from build123d import *

# Parameters (mm, degrees)
BASE_FLANGE1_DEPTH    = 10
FILLET1_R             = 3
SKETCH7_R             = 1.5
SKETCH7_R_2           = 1
CUT_EXTRUDE1_DEPTH    = 39.303728604
BODY_MOVE_COPY1_ANGLE = 90


# Sheet-metal steps are written as plain solids
with BuildPart() as part:
    # Sketch1 → Base-Flange1 (new, symmetric)
    with BuildSketch(Plane.XY):
        with BuildLine():
            Line((-12, 0), (-2.75, 0))
            ThreePointArc((-2.75, 0), (-0.805456352, 0.805456352), (0, 2.75))
            Line((0, 2.75), (0, 15.775))
            ThreePointArc((0, 15.775), (0.219669914, 16.305330086), (0.75, 16.525))
            Line((0.75, 16.525), (32, 16.525))
            Line((32, 16.525), (32, 18.525))
            Line((32, 18.525), (0.75, 18.525))
            ThreePointArc((0.75, 18.525), (-1.194543648, 17.719543648), (-2, 15.775))
            Line((-2, 15.775), (-2, 2.75))
            ThreePointArc((-2, 2.75), (-2.219669914, 2.219669914), (-2.75, 2))
            Line((-2.75, 2), (-12, 2))
            Line((-12, 2), (-12, 0))
        make_face()
    extrude(amount=BASE_FLANGE1_DEPTH, both=True)

    # Fillet1
    fillet1_edges = [part.edges().sort_by_distance(p)[0] for p in [
        (32, 17.525, -10),
        (-12, 1, -10),
        (32, 17.525, 10),
        (-12, 1, 10),
    ]]
    fillet(fillet1_edges, radius=FILLET1_R)

    # Sketch7 → Cut-Extrude1 (cut, through all)
    with BuildSketch(Plane(origin=(0, 0, 0), x_dir=(1, 0, 0), z_dir=(0, 1, 0))):
        with Locations((-9, 6)):
            Circle(SKETCH7_R)
        with Locations((-9, -6)):
            Circle(SKETCH7_R)
        with Locations(Location((14.875, 0, 0), (0, 0, 90))):
            Circle(SKETCH7_R_2)
    extrude(amount=CUT_EXTRUDE1_DEPTH, mode=Mode.SUBTRACT)


with BuildPart() as part_1:
    # Body-Move/Copy1: moved
    add(part.part.rotate(Axis((0, 7.6, 0), (1, 0, 0)), BODY_MOVE_COPY1_ANGLE))


solid = part_1.part
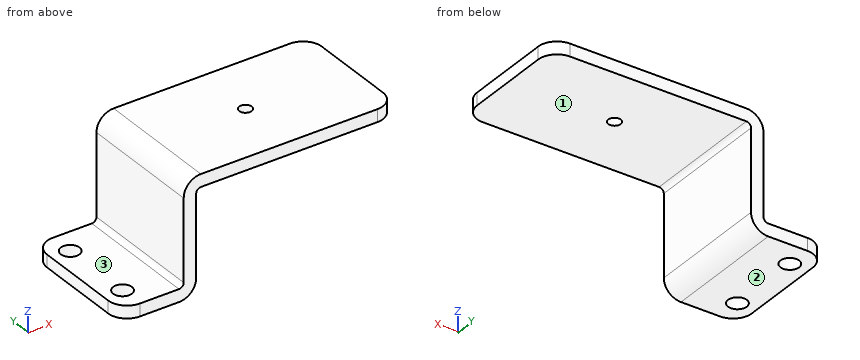
Can you work these out from the model? Positions are in its coordinate system, mm. Face numbers are marked on the shaded views. A direction names the side the tool comes from. Coordinates: 2 decimals unless noted, no trailing zeros. Write each loop counter-clockwise with the first axis right and the second up, starting at its lowest first coordinate (ties: lowest second). Pieces come first, ordered by that corner, then holes.
Q1. For P1, Ø4, axis at x = 22, y = 4, coming from the -Z side (3 decimals); P2, Ø10.5, axis at y = 10.5, z = 0, coming from the -X side; P3, Ø4, axis at y = 6.5, z = 5, coming from the +X side, each with a flat end and sliding along its axis, tell me the tip position at first contact or that it passes through.
Results found:
P1: stops at z = 8.925
P2: stops at x = -2.12
P3: stops at x = 0
Q2. Imagine slicing it at D-D, the plane x = 3. List the corners of the cut face in (y, z) for me (3 decimals).
Results found:
outline: (-2.4, 8.925) - (17.6, 8.925) - (17.6, 10.925) - (-2.4, 10.925) - close
Q3. Please list where these lines run through material, in increasing order: L1, parallel to Y at x = -9, z = -5.95; L2, parallel to X at y = 6.75, z = 0.75; L3, parallel to Z at x = -4, y = 8.
Results found:
L1: y = -2.4 to 0.1, 3.1 to 12.1, 15.1 to 17.6
L2: x = -2 to 0
L3: z = -7.6 to -5.6
Q4. Imagine slicing it at B-B, the plane y = 1.6. List the corners of the cut face in (x, z) for me (3 decimals).
Results found:
outline: (-12, -7.6) - (-10.5, -7.6) - (-10.5, -5.6) - (-12, -5.6) - close; (-7.5, -7.6) - (-2.75, -7.6) arc R2.75 ccw to (0, -4.85) - (0, 8.175) arc R0.75 cw to (0.75, 8.925) - (32, 8.925) - (32, 10.925) - (0.75, 10.925) arc R2.75 ccw to (-2, 8.175) - (-2, -4.85) arc R0.75 cw to (-2.75, -5.6) - (-7.5, -5.6) - close
Q5. Imagine slicing it at C-C, the plane z = 6. List the corners of the cut face in (x, y) for me.
Results found:
outline: (-2, -2.4) - (0, -2.4) - (0, 17.6) - (-2, 17.6) - close
Q6. Imagine slicing it at A-A, the plane y = 7.6. List the corners of the cut face in (x, z) for me (3 decimals).
Results found:
outline: (-12, -7.6) - (-2.75, -7.6) arc R2.75 ccw to (0, -4.85) - (0, 8.175) arc R0.75 cw to (0.75, 8.925) - (13.875, 8.925) - (13.875, 10.925) - (0.75, 10.925) arc R2.75 ccw to (-2, 8.175) - (-2, -4.85) arc R0.75 cw to (-2.75, -5.6) - (-12, -5.6) - close; (15.875, 8.925) - (32, 8.925) - (32, 10.925) - (15.875, 10.925) - close
Q7. Which directions (+Z, -Z, +X, -X, +Y, -Y) give clear straight access to the entire face, cutting with the end or side of a thin tool? Please do the marked faces 1, 2 and 3.
Results found:
face 1: -Z, +X, +Y, -Y
face 2: -Z, +X, -X, +Y, -Y
face 3: +Z, -X, +Y, -Y
